Geometry check sheet. Reference: the model listing, model coordinates, mm. Give positions to 0.01 mm unless a question says otherwise; leave off trailing zeros. Order: outer loops, then holes, each group sorted by start corner. A loop starts at its lowest first (then second) coordinate and runs counter-clockwise, first axis right, second up. Notation, with made-up numbers: M 29.5,-11 L 86.5,-11 A9 cw 86.5,2 Z; hole C 17,79 d10. An arc over 180 degrees is marked long. Answer as CSV lines item,"result".
from build123d import *

# Parameters (mm, degrees)
SKETCH_1_R      = 2
SKETCH_1_R_2    = 1.5
EXTRUDE_2_DEPTH = 5


with BuildPart() as part:
    # 草图1 → 凸台-拉伸2 (new body)
    with BuildSketch(Plane(origin=(0, 0, 0), x_dir=(1, 0, 0), z_dir=(0, 1, 0))):
        with BuildLine():
            Line((-131.385271199, 145), (128.614728801, 145))
            ThreePointArc((128.614728801, 145), (154.115285595, 35), (128.614728801, -75))
            Line((128.614728801, -75), (-131.385271199, -75))
            ThreePointArc((-131.385271199, -75), (-155.884714405, 35), (-131.385271199, 145))
        make_face()
        with Locations(Location((-104.385271199, 118, 0), (0, 0, 270))):
            Circle(SKETCH_1_R, mode=Mode.SUBTRACT)
        with Locations(Location((-118.385271199, 132, 0), (0, 0, 270))):
            Circle(SKETCH_1_R, mode=Mode.SUBTRACT)
        with Locations(Location((-118.385271199, 118, 0), (0, 0, 270))):
            Circle(SKETCH_1_R, mode=Mode.SUBTRACT)
        with Locations(Location((-104.385271199, 132, 0), (0, 0, 270))):
            Circle(SKETCH_1_R, mode=Mode.SUBTRACT)
        with Locations(Location((101.614728801, 132, 0), (0, 0, 270))):
            Circle(SKETCH_1_R, mode=Mode.SUBTRACT)
        with Locations(Location((101.614728801, 118, 0), (0, 0, 270))):
            Circle(SKETCH_1_R, mode=Mode.SUBTRACT)
        with Locations(Location((115.614728801, 118, 0), (0, 0, 270))):
            Circle(SKETCH_1_R, mode=Mode.SUBTRACT)
        with Locations(Location((115.614728801, 132, 0), (0, 0, 270))):
            Circle(SKETCH_1_R, mode=Mode.SUBTRACT)
        with Locations(Location((115.614728801, -45.585551803, 0), (0, 0, 270))):
            Circle(SKETCH_1_R, mode=Mode.SUBTRACT)
        with Locations(Location((115.614728801, -59.585551803, 0), (0, 0, 270))):
            Circle(SKETCH_1_R, mode=Mode.SUBTRACT)
        with Locations(Location((101.614728801, -59.585551803, 0), (0, 0, 270))):
            Circle(SKETCH_1_R, mode=Mode.SUBTRACT)
        with Locations(Location((101.614728801, -45.585551803, 0), (0, 0, 270))):
            Circle(SKETCH_1_R, mode=Mode.SUBTRACT)
        with Locations(Location((-118.385271199, -48, 0), (0, 0, 270))):
            Circle(SKETCH_1_R, mode=Mode.SUBTRACT)
        with Locations(Location((-118.385271199, -62, 0), (0, 0, 270))):
            Circle(SKETCH_1_R, mode=Mode.SUBTRACT)
        with Locations(Location((-104.385271199, -48, 0), (0, 0, 270))):
            Circle(SKETCH_1_R, mode=Mode.SUBTRACT)
        with Locations(Location((-104.385271199, -62, 0), (0, 0, 270))):
            Circle(SKETCH_1_R, mode=Mode.SUBTRACT)
        with Locations(Location((-12.193281543, 35, 0), (0, 0, 270))):
            Circle(SKETCH_1_R_2, mode=Mode.SUBTRACT)
        with Locations(Location((4.806718457, 35, 0), (0, 0, 270))):
            Circle(SKETCH_1_R_2, mode=Mode.SUBTRACT)
        with Locations(Location((-131.385271199, 85, 0), (0, 0, 270))):
            Circle(SKETCH_1_R, mode=Mode.SUBTRACT)
        with Locations(Location((-131.385271199, -15, 0), (0, 0, 270))):
            Circle(SKETCH_1_R, mode=Mode.SUBTRACT)
        with Locations(Location((18.256265761, 70, 0), (0, 0, 270))):
            Circle(SKETCH_1_R, mode=Mode.SUBTRACT)
        with Locations(Location((53.256265761, 70, 0), (0, 0, 270))):
            Circle(SKETCH_1_R, mode=Mode.SUBTRACT)
        with Locations(Location((53.256265761, 0, 0), (0, 0, 270))):
            Circle(SKETCH_1_R, mode=Mode.SUBTRACT)
        with Locations(Location((18.256265761, 0, 0), (0, 0, 270))):
            Circle(SKETCH_1_R, mode=Mode.SUBTRACT)
        with Locations(Location((60.81589639, 55, 0), (0, 0, 270))):
            Circle(SKETCH_1_R, mode=Mode.SUBTRACT)
        with Locations(Location((80.81589639, 55, 0), (0, 0, 270))):
            Circle(SKETCH_1_R, mode=Mode.SUBTRACT)
        with Locations(Location((80.81589639, 15, 0), (0, 0, 270))):
            Circle(SKETCH_1_R, mode=Mode.SUBTRACT)
        with Locations(Location((60.81589639, 15, 0), (0, 0, 270))):
            Circle(SKETCH_1_R, mode=Mode.SUBTRACT)
    extrude(amount=EXTRUDE_2_DEPTH)


solid = part.part
(1) Section check B-B on x = 135. Enter the section's corners in (y, z), then the cut area to 3 significant figures.
The answers:
outline,"M 0,-130.88 L 5,-130.88 L 5,60.88 L 0,60.88 Z"
area,"959 mm2"
(2) Section check C-C on z = 5.5. Enter the section's corners in (x, y), then the cut area to 3 significant figures.
The answers:
outline,"M -152.7,0 L 150.81,0 L 150.81,5 L -152.7,5 Z"
area,"1,520 mm2"
(3) Section check A-A on y = 1.3. State how many separate pieces and enclosed holes the cut face has, then the cut area to 3 significant figures.
The answers:
separate pieces,"1"
enclosed holes,"28"
area,"64,300 mm2"
(4) Gauge pin test, flat end, axial feed: P1, Ø3.5, axis at x = 53.26, z = 0, coming from the -Y side. Record the tip position at first contact, or that the pin passes through.
The answers:
P1,"passes through"
(5) Material ranges on line 1 (X direction, y = 3.95, z = 0); line 2 (Z direction, x = 82, y = 4.6); line 3 (X direction, y = 4, z = -118), recorded low to high.
The answers:
line 1,"x = -153.51 to 16.26, 20.26 to 51.26, 55.26 to 151.65"
line 2,"z = -145 to -56.61, -53.39 to -16.61, -13.39 to 75"
line 3,"x = -142.24 to -120.39, -116.39 to -106.39, -102.39 to 99.61, 103.61 to 113.61, 117.61 to 139.94"
